Part print with two shaded views. Sizes in mm from the minimum x, y, z corner. A direction names the side the tool comes from. Round coordinates to 2 decimals unless told otherwise and drop trailing zeros. Loops run counter-clockwise (first coordinate to the right, second up) from the corner with the lowest first, then second, coordinate; pieces in that order, holes last.
(1) Cut at C-C on y = 104. List the corners of the cut face in (x, z).
(2) Cut at D-D on z = 58.5. List the corners of the cut face in (x, y).
(3) Tool access for the marked faces 4 and 5: list every direction of +Z, -Z, +X, -X, +Y, -Y with a clear straight run to the whole face (end or side of a thin tool).
(4) Mould opens along X. For the marked faces 1, 2 and 3 say: +X half, -X half, draft (parallel to the pull), parting line (faces both ways), or undercut.
(5) Flat gauge pin, fed straight in: pin 1 (10 mm diameter, centred on x = 42.5, z = 57, fed in from +Y). Where does the tip first touch, or does it go through?
(6) Cut at B-B on x = 69.85. List the corners of the cut face in (y, z) (3 decimals).
(7) Probe probe 1 along X at (y, z) = (67.5, 117); probe 2 along Z at (x, y) = (85, 91); probe 3 along Y at (x, z) = (69.85, 134) (3 decimals). List the from-to ranges inside material, lowest first.
(8) Cut at A-A on y = 88.9. List the corners of the cut face in (x, z).
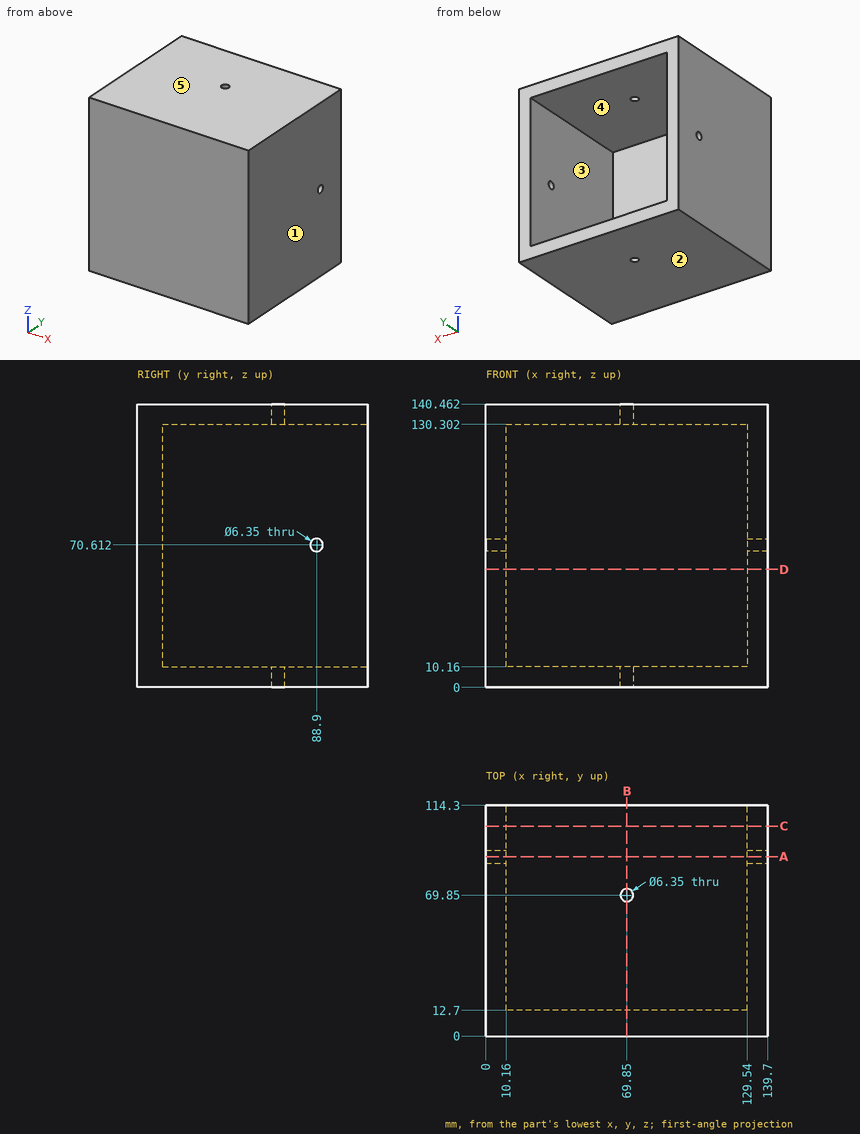
Final values:
1. outline: (0, 0) - (139.7, 0) - (139.7, 140.46) - (0, 140.46) - close; hole (10.16, 10.16) - (129.54, 10.16) - (129.54, 130.3) - (10.16, 130.3) - close
2. outline: (0, 0) - (139.7, 0) - (139.7, 114.3) - (129.54, 114.3) - (129.54, 12.7) - (10.16, 12.7) - (10.16, 114.3) - (0, 114.3) - close
3. face 4: +Y
3. face 5: +Z, +X, -X, +Y, -Y
4. face 1: +X half
4. face 2: draft
4. face 3: undercut
5. pin 1: stops at y = 12.7
6. outline: (0, 0) - (66.675, 0) - (66.675, 10.16) - (12.7, 10.16) - (12.7, 130.302) - (66.675, 130.302) - (66.675, 140.462) - (0, 140.462) - close; (73.025, 0) - (114.3, 0) - (114.3, 10.16) - (73.025, 10.16) - close; (73.025, 130.302) - (114.3, 130.302) - (114.3, 140.462) - (73.025, 140.462) - close
7. probe 1: x = 0 to 10.16, 129.54 to 139.7
7. probe 2: z = 0 to 10.16, 130.3 to 140.46
7. probe 3: y = 0 to 66.675, 73.025 to 114.3
8. outline: (0, 0) - (139.7, 0) - (139.7, 67.44) - (129.54, 67.44) - (129.54, 10.16) - (10.16, 10.16) - (10.16, 67.44) - (0, 67.44) - close; (0, 73.79) - (10.16, 73.79) - (10.16, 130.3) - (129.54, 130.3) - (129.54, 73.79) - (139.7, 73.79) - (139.7, 140.46) - (0, 140.46) - close
